```python
from build123d import *


with BuildPart() as part:
    # Sketch1 → Revolve5 (revolve)
    with BuildSketch(Plane.XY, mode=Mode.PRIVATE) as revolve5_sk:
        with BuildLine():
            Line((0, 7), (3.5, 7))
            Line((3.5, 7), (3.5, 6.5))
            Line((3.5, 6.5), (0.5, 6.5))
            Line((0.5, 6.5), (0.5, 5.5))
            Line((0.5, 5.5), (1.691723883, 5.026212332))
            ThreePointArc((1.691723883, 5.026212332), (2.270416983, 6.065978794), (1.977233578, 4.912703679))
            Line((1.977233578, 4.912703679), (2.17265883, 4.835009445))
            Line((2.17265883, 4.835009445), (2.823645607, 5.3))
            Line((2.823645607, 5.3), (2.9, 5))
            Line((2.9, 5), (2.9, 4.5))
            Line((2.9, 4.5), (2.8, 4.5))
            Line((2.8, 4.5), (2.8, 4.928571429))
            Line((2.8, 4.928571429), (2.2, 4.5))
            Line((2.2, 4.5), (0, 5.35))
            Line((0, 5.35), (0, 7))
        make_face()
    revolve(revolve5_sk.sketch.rotate(Axis((0, 0, 0), (1, 0, 0)), 90), axis=Axis((0, 0, 0), (1, 0, 0)))


solid = part.part
```
Verification items for the finished model (mm, model axes). A direction names the side the tool comes from. Give positions to 0.01 mm unless a question says otherwise; leave off trailing zeros. Order: outer loops, then holes, each group sorted by start corner. A loop starts at its lowest first (then second) coordinate and runs counter-clockwise, first axis right, second up. Notation, with made-up numbers: (26, 23.25) -> (38, 23.25) arc R24 cw to (38, 61.25) -> close; hole circle Ø11 at (18.5, -12). An arc over 180 degrees is marked (long way). One line per item, written item: value.
(1) Scan lines: line 1 along Z through (x, y) = (1.3, -4.25); line 2 along Y through (x, z) = (1, -4); line 3 along Y through (x, z) = (1.85, 0). Record each from-to range of solid material in increasing order. Write a range as [from, to].
Final values:
line 1: [-5.56, -4.92], [-2.96, -2.33], [2.33, 2.96], [4.92, 5.56]
line 2: [-5.74, -5.12], [-3.48, -2.94], [2.94, 3.48], [5.12, 5.74]
line 3: [-7, -6.5], [-6.07, -4.64], [4.64, 6.07], [6.5, 7]
(2) Sectioned sample at C-C on x = 1.15. Record the cut outline in (y, z), then the cut area to 3 significant figures.
Final values:
outline: circle Ø14 at (0, 0); circle Ø10.48 at (0, 0); hole circle Ø13 at (0, 0); hole circle Ø9.81 at (0, 0)
area: 31.9 mm^2
(3) Draft check along Y on faces 1 (the face through (1.77, 6.21, 3.23)), 2 (the face through (2.06, -0.2, -4.55)), 3 (the face through (0, 3, 5)). Enter one of: pulls with the +Y half, pulls with the -Y half, needs draft (parallel to the pull), parting line crosses it, or undercut.
Final values:
face 1: parting line crosses it
face 2: undercut
face 3: needs draft
(4) Tool access check on faces 4 (the face through (0.5, -3, -5)), 5 (the face through (1.979, 3.955, -5.158)). Record the directions out of +Z, -Z, +X, -X, +Y, -Y that give a thin tool (end or side, any length) a straight path to the whole face; none if there is none.
Final values:
face 4: none
face 5: +X
(5) Gauge pin test, flat ends, axial feed: pin 1 (5 mm diameter, centred on y = -2.5, z = -1, fed in from +X); pin 2 (1.5 mm diameter, centred on x = 2, z = -3, fed in from +Y). Record the tip position at first contact, or that the pin passes through.
Final values:
pin 1: x = 2.9
pin 2: y = 6.63
